Read the model definition and answer for the solid it produces. Units are mm, in the model's axes. A direction names the side the tool comes from. Give positions to 0.01 mm unless a question says otherwise; leave off trailing zeros. Order: outer loops, then holes, each group sorted by start corner. A loop starts at its lowest first (then second) coordinate and runs counter-clockwise, first axis right, second up. Notation, with made-up numbers: (67, 21) -> (117, 21) arc R11 ccw to (117, 37) -> close; hole circle Ø5 at (-6, 56). An arc over 180 degrees is marked (long way). Answer as CSV lines item,"result". Start each with the question number.
1) For faces 4 (the face through (7.51, 0.44, 0.74)), 5 (the face through (12.6, 1.92, 0.74)), determine the directions among +Z, -Z, +X, -X, +Y, -Y from which every point of the face is accessible in a straight line to the end or side of a thin tool.
2) A flat-ended cylindrical pin translates along its axis: pin 1 Ø1 at (x, y) = (8, 1.5) entering from -Z. Find the tip coordinate at first contact, or state that the pin passes through.
3) Find section A-A (y = 2). Determine the outline of the cut face in (x, z).
4) Straight lines are drawn through the part: L1, parallel to X at y = -0.5, z = 1.2; L2, parallel to X at y = -1, z = 1.3; L3, parallel to X at y = 1.75, z = 1.2. For each, find the intervals that lie inside material, in ascending order. Write a range as from..to.
5) The mould has two halves that part along X. Classify faces 1 (the face through (5, -1, 1.5)), 2 (the face through (5.6, -5, 0.7)), 3 (the face through (9.75, -0.05, 0.74)): +X half, -X half, draft (parallel to the pull), parting line (faces both ways), or undercut.
6) Find section C-C (x = 11). Determine the outline of the cut face in (y, z), and give its area (3 significant figures).
7) Find section D-D (y = 0.75). Determine the outline of the cut face in (x, z), and give its area (3 significant figures).
Autodesk Inventor part; units mm, degrees
ref_plane "YZ Plane" through (0, 0, 0) normal (1, 0, 0) x (0, 1, 0)
ref_plane "XZ Plane" through (0, 0, 0) normal (0, 1, 0) x (-1, 0, 0)
ref_plane "XY Plane" through (0, 0, 0) normal (0, 0, 1) x (1, 0, 0)
sketch "Sketch1" plane through (0, 0, 0) normal (0, 0, 1) x (1, 0, 0)
  circle A0 centre (0, 0) radius 1.25
  line L0 (0, 0) -> (11, 0) construction
  circle A1 centre (11, 0) radius 1.25
  arc A2 (1.8836, 1.6438) -> (-1.8836, -1.6438) centre (0, 0) ccw
  arc A3 (12.8836, -1.6438) -> (9.1164, 1.6438) centre (11, 0) ccw
  arc A4 (-1.8836, -1.6438) -> (12.8836, -1.6438) centre (5.5, 4.8) ccw
  arc A5 (1.8836, 1.6438) -> (5.5, 0) centre (5.5, 4.8) ccw
  arc A6 (5.5, 0) -> (9.1164, 1.6438) centre (5.5, 4.8) ccw
  dimension "d0" = 2.5
  dimension "d1" = 11
  dimension "d8" = 5
extrude "Extrusion1" add sketch "Sketch1" along normal blind 1.5
properties part number "linkageC"
Findings below:
1,face 4,"+Z, -Z, +Y"
1,face 5,"+Z, -Z"
2,pin 1,"through"
3,outline,"(-1.5, 0) -> (1.5, 0) -> (1.5, 1.5) -> (-1.5, 1.5) -> close; (9.5, 0) -> (12.5, 0) -> (12.5, 1.5) -> (9.5, 1.5) -> close"
4,L1,"-2.45..-1.15, 1.15..9.85, 12.15..13.45"
4,L2,"-2.29..-0.75, 0.75..10.25, 11.75..13.29"
4,L3,"-1.79..1.79, 9.21..12.79"
5,face 1,"draft"
5,face 2,"parting line"
5,face 3,"undercut"
6,outline,"(-3.31, 0) -> (-1.25, 0) -> (-1.25, 1.5) -> (-3.31, 1.5) -> close; (1.25, 0) -> (2.5, 0) -> (2.5, 1.5) -> (1.25, 1.5) -> close"
6,area,"4.97 mm²"
7,outline,"(-2.38, 0) -> (-1, 0) -> (-1, 1.5) -> (-2.38, 1.5) -> close; (1, 0) -> (2.92, 0) -> (2.92, 1.5) -> (1, 1.5) -> close; (8.08, 0) -> (10, 0) -> (10, 1.5) -> (8.08, 1.5) -> close; (12, 0) -> (13.38, 0) -> (13.38, 1.5) -> (12, 1.5) -> close"
7,area,"9.93 mm²"
